```python
from build123d import *

# Parameters (mm, degrees)
BOSS_EXTRUDE1_DEPTH  = 20
SKETCH3_W            = 12
SKETCH3_H            = 20
BOSS_EXTRUDE2_DEPTH  = 5
FILLET1_R            = 6
FILLET2_R            = 3
SKETCH4_R            = 2
CUT_EXTRUDE1_DEPTH   = 6
SKETCH5_W            = 2
SKETCH5_H            = 20
SKETCH5_W_2          = 3
BOSS_EXTRUDE3_DEPTH  = 4
SKETCH6_W            = 2
SKETCH6_H            = 20
BOSS_EXTRUDE4_DEPTH  = 3
SKETCH7_W            = 2
SKETCH7_H            = 20
BOSS_EXTRUDE5_DEPTH  = 7
FILLET3_R            = 3
SKETCH8_W            = 18
SKETCH8_H            = 22
BOSS_EXTRUDE6_DEPTH  = 5
CUT_EXTRUDE2_START   = -4
CUT_EXTRUDE2_DEPTH   = 40.285832851
CUT_EXTRUDE3_DEPTH   = 36.285832851
FILLET4_R            = 3
SKETCH11_W           = 18
SKETCH11_H           = 22
CUT_EXTRUDE4_DEPTH   = 1
FILLET5_R            = 3
FILLET4_OF_MIRROR1_R = 3
SKETCH12_W           = 16.003556493
SKETCH12_H           = 33.094462643
CUT_EXTRUDE5_DEPTH   = 22


with BuildPart() as part:
    # Sketch1 → Boss-Extrude1 (new body)
    with BuildSketch(Plane(origin=(0, 0, 0), x_dir=(1, 0, 0), z_dir=(0, 1, 0))):
        with BuildLine():
            Line((0, 15.3), (0, -12.3))
            ThreePointArc((0, -12.3), (-2, -14.3), (-4, -12.3))
            Line((-4, -12.3), (-7, -12.3))
            Line((-7, -12.3), (-7, -17.3))
            Line((-7, -17.3), (5, -17.3))
            Line((5, -17.3), (5, 20.3))
            Line((5, 20.3), (-7, 20.3))
            Line((-7, 20.3), (-7, 15.3))
            Line((-7, 15.3), (-4, 15.3))
            ThreePointArc((-4, 15.3), (-2, 17.3), (0, 15.3))
        make_face()
    extrude(amount=BOSS_EXTRUDE1_DEPTH)

    # Sketch3 → Boss-Extrude2 (add)
    with BuildSketch(Plane(origin=(0, 0, -20.3), x_dir=(-1, 0, 0), z_dir=(0, 0, -1))):
        with Locations((1, 10)):
            Rectangle(SKETCH3_W, SKETCH3_H)
    extrude(amount=BOSS_EXTRUDE2_DEPTH)

    # Fillet1
    fillet1_edges = [part.edges().sort_by_distance(p)[0] for p in [
        (5, 10, 17.3),
    ]]
    fillet(fillet1_edges, radius=FILLET1_R)

    # Fillet2
    fillet2_edges = [part.edges().sort_by_distance(p)[0] for p in [
        (5, 10, -25.3),
    ]]
    fillet(fillet2_edges, radius=FILLET2_R)

    # Sketch4 → Cut-Extrude1 (cut)
    with BuildSketch(Plane(origin=(0, 0, -25.3), x_dir=(-1, 0, 0), z_dir=(0, 0, -1))):
        with Locations((0.5, 10)):
            Circle(SKETCH4_R)
    extrude(amount=-CUT_EXTRUDE1_DEPTH, mode=Mode.SUBTRACT)

    # Sketch5 → Boss-Extrude3 (add)
    with BuildSketch(Plane.ZY.offset(7)):
        with Locations((16.3, 10)):
            Rectangle(SKETCH5_W, SKETCH5_H)
        with Locations((-23.8, 10)):
            Rectangle(SKETCH5_W_2, SKETCH5_H)
    extrude(amount=BOSS_EXTRUDE3_DEPTH)

    # Sketch6 → Boss-Extrude4 (add)
    with BuildSketch(Plane(origin=(0, 0, 15.3), x_dir=(-1, 0, 0), z_dir=(0, 0, -1))):
        with Locations((10, 10)):
            Rectangle(SKETCH6_W, SKETCH6_H)
    extrude(amount=BOSS_EXTRUDE4_DEPTH)

    # Sketch7 → Boss-Extrude5 (add)
    with BuildSketch(Plane.XY.offset(-22.3)):
        with Locations((-10, 10)):
            Rectangle(SKETCH7_W, SKETCH7_H)
    extrude(amount=BOSS_EXTRUDE5_DEPTH)

    # Fillet3
    fillet3_edges = [part.edges().sort_by_distance(p)[0] for p in [
        (-11, 10, 17.3),
        (-11, 10, -25.3),
    ]]
    fillet(fillet3_edges, radius=FILLET3_R)

    # Sketch8 → Boss-Extrude6 (add)
    with BuildSketch(Plane.ZY):
        with Locations((-6.3, -11)):
            Rectangle(SKETCH8_W, SKETCH8_H)
    boss_extrude6 = extrude(amount=-BOSS_EXTRUDE6_DEPTH)

    # Sketch9 → Cut-Extrude2 (cut)
    with BuildSketch(Plane.ZY.offset(CUT_EXTRUDE2_START)):
        with BuildLine():
            Line((2.7, -10.2), (2.7, -7.2))
            ThreePointArc((2.7, -7.2), (-7.835653753, -11.522921748), (-12.298666607, -22))
            Line((-12.298666607, -22), (-9.298333218, -22))
            ThreePointArc((-9.298333218, -22), (-5.714273587, -13.644300146), (2.7, -10.2))
        make_face()
    cut_extrude2 = extrude(amount=CUT_EXTRUDE2_DEPTH, mode=Mode.SUBTRACT)

    # Sketch9<3> → Cut-Extrude3 (cut, symmetric)
    with BuildSketch(Plane.ZY):
        with BuildLine():
            Line((2.7, -22), (2.7, -10.2))
            ThreePointArc((2.7, -10.2), (-5.714273587, -13.644300146), (-9.298333218, -22))
            Line((-9.298333218, -22), (2.7, -22))
        make_face()
    cut_extrude3 = extrude(amount=CUT_EXTRUDE3_DEPTH, both=True, mode=Mode.SUBTRACT)

    # Fillet4
    fillet4_edges = [part.edges().sort_by_distance(p)[0] for p in [
        (4, -11.522921748, -7.835653753),
    ]]
    fillet(fillet4_edges, radius=FILLET4_R - 0.0001)  # a hair under: the kernel refuses the full size

    # Sketch11 → Cut-Extrude4 (cut)
    with BuildSketch(Plane.ZY):
        with Locations((-6.3, -11)):
            Rectangle(SKETCH11_W, SKETCH11_H)
    cut_extrude4 = extrude(amount=-CUT_EXTRUDE4_DEPTH, mode=Mode.SUBTRACT)

    # Fillet5
    fillet5_edges = [part.edges().sort_by_distance(p)[0] for p in [
        (3, 0, -15.3),
        (3, 0, 2.7),
    ]]
    fillet(fillet5_edges, radius=FILLET5_R)

    # Mirror1: Boss-Extrude6, Cut-Extrude2, Cut-Extrude3, Cut-Extrude4 across plane
    add(boss_extrude6.mirror(Plane(origin=(0, 10, 0), x_dir=(0, 0, 1), z_dir=(0, -1, 0))))
    add(cut_extrude2.mirror(Plane(origin=(0, 10, 0), x_dir=(0, 0, 1), z_dir=(0, -1, 0))), mode=Mode.SUBTRACT)
    add(cut_extrude3.mirror(Plane(origin=(0, 10, 0), x_dir=(0, 0, 1), z_dir=(0, -1, 0))), mode=Mode.SUBTRACT)
    add(cut_extrude4.mirror(Plane(origin=(0, 10, 0), x_dir=(0, 0, 1), z_dir=(0, -1, 0))), mode=Mode.SUBTRACT)

    # Fillet4 of Mirror1
    fillet4_of_mirror1_edges = [part.edges().sort_by_distance(p)[0] for p in [
        (4, 31.522921748, -7.835653753),
    ]]
    fillet(fillet4_of_mirror1_edges, radius=FILLET4_OF_MIRROR1_R - 0.0001)  # a hair under: the kernel refuses the full size

    # Sketch12 → Cut-Extrude5 (cut)
    with BuildSketch(Plane.XZ.offset(22)):
        with Locations((1.208141139, -2.187750571)):
            Rectangle(SKETCH12_W, SKETCH12_H)
    extrude(amount=-CUT_EXTRUDE5_DEPTH, mode=Mode.SUBTRACT)


solid = part.part
```
Part model, mm, in its own coordinate system. A direction names the side the tool comes from. Coordinates: 2 decimals unless noted, no trailing zeros. Order: outer loops, then holes, each group sorted by start corner. A loop starts at its lowest first (then second) coordinate and runs counter-clockwise, first axis right, second up. Notation, with made-up numbers: (57.25, 81) - (104.25, 81) arc R37 ccw to (104.25, 118) - close; hole circle Ø3 at (-38.75, 29). An arc over 180 degrees is marked (long way). Return JSON: item names as keys, results as strings. Group by question number.
Item 1: Cut at B-B (z = -13.5). List the corners of the cut face in (x, y), plus the area to 3 significant figures.
Item 2: Pull direction X, two halves, no side cores. Call faces 1 (the face through (-10, 10, 12.3)), 2 (the face through (-11, 10, -19)), 3 (the face through (-0.24, 11.983, -22.342)): pulls with the +X half, pulls with the -X half, needs draft (parallel to the pull), parting line crosses it, or undercut.
Item 3: Drill centre lines: probe 1 along Z at (x, y) = (-8, 15.5); probe 2 along Y at (x, z) = (-0.5, -23.25); probe 3 along Z at (x, y) = (-6, 14). Where is each one in solid material? Low to high. Write a range as from..to.
Item 4: Which spindle directions (+Z, -Z, +X, -X, +Y, -Y) get a long thin tool onto all of the face, cutting with end or side? Do faces 4 (the face through (-9, 10, -19)), 5 (the face through (-5, 10, 12.3)), 6 (the face through (0, 10, -19.3)). Say none if no direction does.
Item 5: Cut at A-A (y = 10). List the corners of the cut face in (x, z).
Item 6: Cut at D-D (x = 3.25). List the corners of the cut face in (y, z), plus the area to 3 significant figures.
Item 7: Cut at C-C (x = -2). List the corners of the cut face in (y, z).
Item 8: Pin check, flat tips, straight feed: pin 1 (5.5 mm diameter, centred on y = 34.5, z = -6.5, fed in from -X); pin 2 (8 mm diameter, centred on y = 17, z = 3, fed in from -X); pin 3 (3.5 mm diameter, centred on x = -0.5, y = 10, fed in from -Z); pin 4 (6 mm diameter, centred on y = 36.5, z = -1, fed in from -X). Stop position of each tip, or through.
Check values:
{
 "1": {"outline": "(0, 0) - (5, 0) - (5, 42) - (1, 42) - (1, 20) - (0, 20) - close", "area": "188 mm2"},
 "2": {"face 1": "needs draft", "face 2": "pulls with the -X half", "face 3": "undercut"},
 "3": {"probe 1": "z = -25.3..-22.3, 15.3..17.3", "probe 2": "y = 0..8, 12..20", "probe 3": "z = -25.3..-15.3, 12.3..17.3"},
 "4": {"face 4": "+Y, -Y", "face 5": "-X, +Y, -Y", "face 6": "-Z"},
 "5": {"outline": "(-11, -22.3) arc R3 ccw to (-8, -25.3) - (-2.5, -25.3) - (-2.5, -19.3) - (1.5, -19.3) - (1.5, -25.3) - (2, -25.3) arc R3 ccw to (5, -22.3) - (5, 11.3) arc R6 ccw to (-1, 17.3) - (-8, 17.3) arc R3 ccw to (-11, 14.3) - (-11, 12.3) - (-9, 12.3) - (-9, 15.3) - (-7, 15.3) - (-7, 12.3) - (-4, 12.3) arc R2 cw to (0, 12.3) - (0, -15.3) arc R2 cw to (-4, -15.3) - (-7, -15.3) - (-7, -22.3) - (-9, -22.3) - (-9, -15.3) - (-11, -15.3) - close"},
 "6": {"outline": "(0, -25.03) - (20, -25.03) - (20, -15.3) - (42, -15.3) - (42, -11.28) arc R13.98 cw to (28.22, 2.7) - (20, 2.7) - (20, 15.54) - (0, 15.54) - close", "area": "1,060 mm2"},
 "7": {"outline": "(0, -25.3) - (8.68, -25.3) - (8.68, -19.3) - (11.32, -19.3) - (11.32, -25.3) - (20, -25.3) - (20, -17.3) - (0, -17.3) - close; (0, 14.3) - (20, 14.3) - (20, 17.3) - (0, 17.3) - close"},
 "8": {"pin 1": "stops at x = 2.21", "pin 2": "stops at x = 0", "pin 3": "stops at z = -19.3", "pin 4": "passes through"}
}
